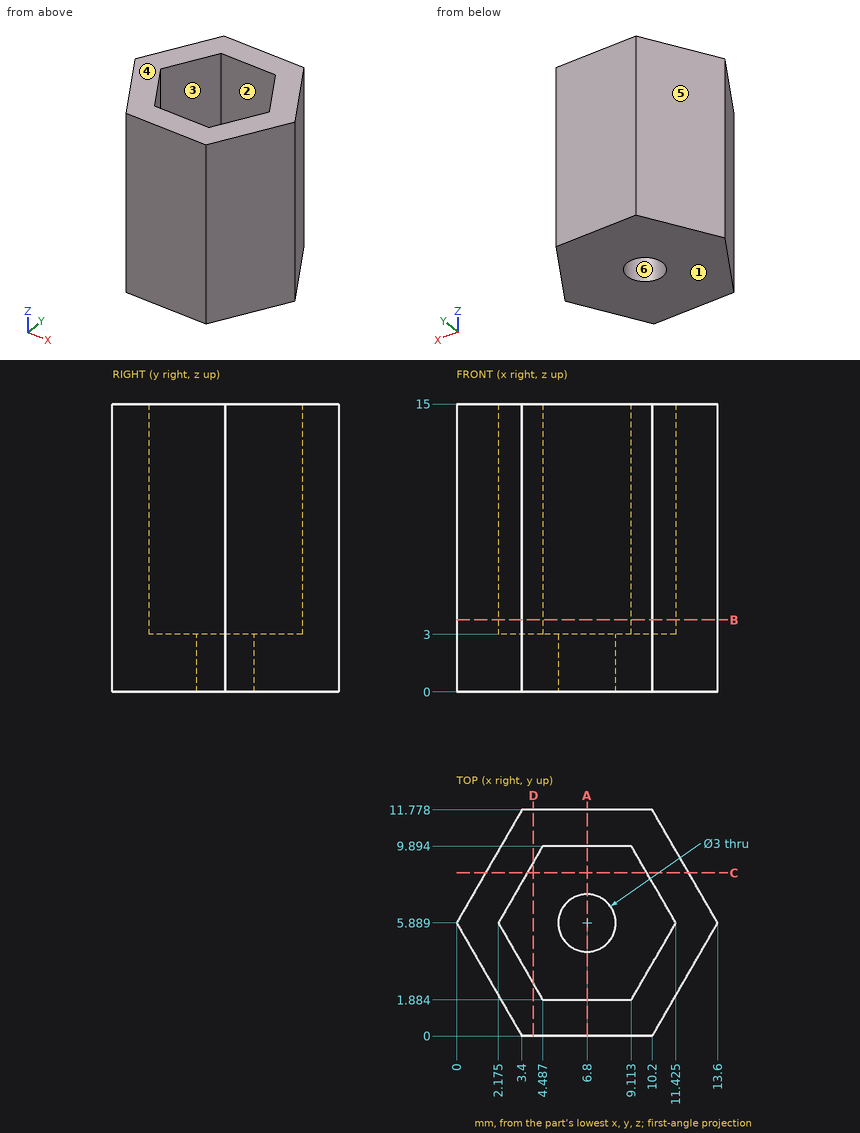
Source: three-view drawing plus pictorial views. Frame: mm from the lowest corner of the part. A direction names the side the tool comes from. Round coordinates to 2 decimals unless told otherwise and drop trailing zeros. Loops run counter-clockwise (first coordinate to the right, second up) from the corner with the lowest first, then second, coordinate; pieces in that order, holes last. Notation, with made-up numbers: (5, -30.75) - (40, -30.75) arc R29 ccw to (40, 0.25) - close; hole circle Ø9 at (-2.75, 41). An arc over 180 degrees is marked (long way). Write item = value, one per line. Start each with the question number.
Item 1: Material intervals for line 1 (Y direction, x = 6.8, z = 1.4); line 2 (Y direction, x = 5.25, z = 8.5) (1 decimal); line 3 (Z direction, x = 5.5, y = 8.5), sorted ascending.
Item 2: Mould query, pull axis Y, two halves, no side actions, for the marked faces 3, 4, 5 and 6. Classes: released by +Y, released by -Y, zero draft, split by the parting line, or undercut.
Item 3: Section query C-C on y = 8.5. Output: boundary loops of the cut face in (x, z).
Item 4: First-contact query: pin 1 Ø2.5 at (x, y) = (7.5, 7) entering from +Z; pin 2 Ø5 at (y, z) = (10, 5.5) entering from +X. Flat tips, straight axial feed; report the tip coordinate or a pass-through.
Item 5: Section query D-D on x = 4. Output: boundary loops of the cut face in (y, z).
Item 6: Section query A-A on x = 6.8. Output: boundary loops of the cut face in (y, z) (1 decimal).
Item 7: Reachability of the marked faces 1 and 2 from +Z, -Z, +X, -X, +Y, -Y: full face, straight path, thin tool, end or side. Return the list, or none.
Item 8: Section query B-B on z = 3.75. Output: boundary loops of the cut face in (x, y) (1 decimal).
Results list:
q1.line_1 = 0 to 4.39, 7.39 to 11.78
q1.line_2 = 0 to 1.9, 9.9 to 11.8
q1.line_3 = 0 to 3
q2.face_3 = undercut
q2.face_4 = zero draft
q2.face_5 = released by +Y
q2.face_6 = undercut
q3.outline = (1.51, 0) - (12.09, 0) - (12.09, 15) - (9.92, 15) - (9.92, 3) - (3.68, 3) - (3.68, 15) - (1.51, 15) - close
q4.pin_1 = 3
q4.pin_2 = 12.67
q5.outline = (0, 0) - (11.78, 0) - (11.78, 15) - (9.05, 15) - (9.05, 3) - (2.73, 3) - (2.73, 15) - (0, 15) - close
q6.outline = (0, 0) - (4.4, 0) - (4.4, 3) - (1.9, 3) - (1.9, 15) - (0, 15) - close; (7.4, 0) - (11.8, 0) - (11.8, 15) - (9.9, 15) - (9.9, 3) - (7.4, 3) - close
q7.face_1 = -Z, +X, -X, +Y, -Y
q7.face_2 = +Z
q8.outline = (0, 5.9) - (3.4, 0) - (10.2, 0) - (13.6, 5.9) - (10.2, 11.8) - (3.4, 11.8) - close; hole (2.2, 5.9) - (4.5, 1.9) - (9.1, 1.9) - (11.4, 5.9) - (9.1, 9.9) - (4.5, 9.9) - close
